Here's how the part is built. I have some questions about the finished solid (model axes, mm). Face numbers are marked on the shaded views. Round coordinates to 2 decimals unless told otherwise and drop trailing zeros. Loops run counter-clockwise (first coordinate to the right, second up) from the corner with the lowest first, then second, coordinate; pieces in that order, holes last. Notation, with made-up numbers: M 66,47 L 88,47 A27 cw 88,78 Z; hole C 26,10 d7. An arc over 180 degrees is marked long. Use a Markdown table: item, result.
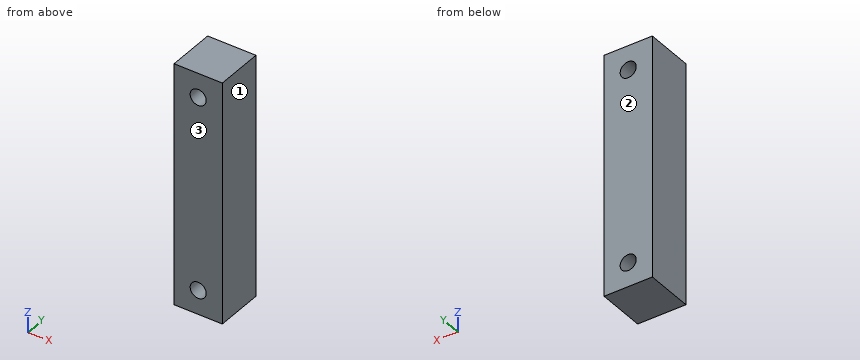
Autodesk Inventor part; units mm, degrees
ref_plane "YZ Plane" through (0, 0, 0) normal (1, 0, 0) x (0, 1, 0)
ref_plane "XZ Plane" through (0, 0, 0) normal (0, 1, 0) x (-1, 0, 0)
ref_plane "XY Plane" through (0, 0, 0) normal (0, 0, 1) x (1, 0, 0)
sketch "スケッチ4" plane through (0, 0, 0) normal (0, 0, 1) x (1, 0, 0)
  line L0 (-15, 15) -> (15, 15)
  line L1 (15, 15) -> (15, -15)
  line L2 (15, -15) -> (-15, -15)
  line L3 (-15, -15) -> (-15, 15)
  line L4 (-15, 15) -> (15, -15) construction
  line L5 (15, 15) -> (-15, -15) construction
  point P0 (0, 0)
  dimension "d14" = 30
  dimension "d15" = 30
extrude "押し出し2" add sketch "スケッチ4" along normal blind 150.185
sketch "スケッチ5" plane through (-15, 15, 0) normal (0, 1, 0) x (1, 0, 0)
  line L0 (30, -150.185) -> (0, -150.185)
  line L1 (0, 0) -> (30, 0)
  point P0 (15, 0)
  point P1 (15, -135.185)
  point P2 (15, -15)
  dimension "d18" = 15
  dimension "d19" = 15
hole "穴2" at (0, 15, 135.185) at (0, 15, 15) direction (0, -1, 0) diameter 10 end through all
Q1. Imagine slicing it at D-D, the plane z = 138.5. Please give me the cut outline in (x, y), then the cut area to 3 significant figures.
Return value:
| item | result |
|---|---|
| outline | M -15,-15 L -3.74,-15 L -3.74,15 L -15,15 Z; M 3.74,-15 L 15,-15 L 15,15 L 3.74,15 Z |
| area | 675 mm^2 |
Q2. I need wall thicknesses on line 1 (Z direction, x = 0, y = 2.5) (3 decimals); line 2 (X direction, y = 6.5, z = 15); line 3 (Z direction, x = -2.25, y = 11.75) (3 decimals). Which ranges of each line are inside material? Lowest first, please. Write a range as from..to.
Return value:
| item | result |
|---|---|
| line 1 | z = 0..10, 20..130.185, 140.185..150.185 |
| line 2 | x = -15..-5, 5..15 |
| line 3 | z = 0..10.535, 19.465..130.72, 139.65..150.185 |
Q3. Imagine slicing it at C-C, the plane y = 0.5. Please give me the cut outline in (x, z) (3 decimals).
Return value:
| item | result |
|---|---|
| outline | M -15,0 L 15,0 L 15,150.185 L -15,150.185 Z; hole C 0,15 d10; hole C 0,135.185 d10 |
Q4. Imagine slicing it at B-B, the plane x = 0. Please give me the cut outline in (y, z) (3 decimals).
Return value:
| item | result |
|---|---|
| outline | M -15,0 L 15,0 L 15,10 L -15,10 Z; M -15,20 L 15,20 L 15,130.185 L -15,130.185 Z; M -15,140.185 L 15,140.185 L 15,150.185 L -15,150.185 Z |
Q5. We'd pull the mould along Y, two halves only. Please class the marked faces 1, 2 and 3: pulls with the +Y half, pulls with the -Y half, needs draft (parallel to the pull), parting line crosses it, or undercut.
Return value:
| item | result |
|---|---|
| face 1 | needs draft |
| face 2 | pulls with the +Y half |
| face 3 | pulls with the -Y half |
Q6. Will this pin go through, and if not, where does the flat tip stop? P1, Ø12, axis at x = 3.5, y = -5.5, coming from the -Z side.
Return value:
| item | result |
|---|---|
| P1 | stops at z = 0 |
Q7. Imagine slicing it at A-A, the plane z = 15. Please give me the cut outline in (x, y).
Return value:
| item | result |
|---|---|
| outline | M -15,-15 L -5,-15 L -5,15 L -15,15 Z; M 5,-15 L 15,-15 L 15,15 L 5,15 Z |
